Work out the finished part from the listing and answer in its coordinate system (mm). A direction names the side the tool comes from. Round coordinates to 2 decimals unless told otherwise and drop trailing zeros. Write each loop counter-clockwise with the first axis right and the second up, starting at its lowest first coordinate (ties: lowest second). Pieces come first, ordered by that corner, then holes. Notation, with made-up numbers: (-24, 84.25) - (-3, 84.25) arc R33 cw to (-3, 117.25) - close; hole circle Ø6 at (65.5, 21.25). An arc over 180 degrees is marked (long way). Answer as a JSON object with one key per item and string values.
```python
from build123d import *

# Parameters (mm, degrees)
BOSS_EXTRUDE1_DEPTH     = 640
BOSS_EXTRUDE2_DEPTH     = 63
BOSS_EXTRUDE3_DEPTH     = 7
SKETCH26_R              = 6
CUT_EXTRUDE2_DEPTH      = 10
CUT_EXTRUDE1_DEPTH      = 10
CUT_EXTRUDE1_DEPTH_BACK = 10
SKETCH28_R              = 6


with BuildPart() as part:
    # Sketch1 → Boss-Extrude1 (new body)
    with BuildSketch(Plane.XY):
        Polygon((0, 0), (0, 70), (70, 70), (70, 63), (7, 63), (7, 0), align=None)
    extrude(amount=BOSS_EXTRUDE1_DEPTH)

    # Sketch23 → Boss-Extrude2 (add)
    with BuildSketch(Plane(origin=(0, 0, 0), x_dir=(1, 0, 0), z_dir=(0, 1, 0))):
        Polygon((0, -640), (42.5, -713.612159322), (48.562177826, -710.112159322), (7, -640), align=None)
    extrude(amount=BOSS_EXTRUDE2_DEPTH)

    # Sketch25 → Boss-Extrude3 (add)
    with BuildSketch(Plane(origin=(0, 63, 0), x_dir=(1, 0, 0), z_dir=(0, 1, 0))):
        Polygon((70, -640), (0, -640), (42.5, -713.612159322), (70, -713.612159322), align=None)
    extrude(amount=BOSS_EXTRUDE3_DEPTH)

    # Sketch26 → Cut-Extrude2 (cut)
    with BuildSketch(Plane(origin=(-275.556719825, 0, 163.348804279), x_dir=(-0.5099316128113042, 0, -0.8602149442178172), z_dir=(0.8602149442178172, 0, -0.5099316128113042))):
        with Locations((-614.36248118, 31.5)):
            Circle(SKETCH26_R)
        with Locations((-575.357085589, 31.5)):
            Circle(SKETCH26_R)
    extrude(amount=-CUT_EXTRUDE2_DEPTH, mode=Mode.SUBTRACT)

    # Mirror1: part across plane


with BuildPart() as part_1:
    add(part.part)
    add(part.part.mirror(Plane.XY))

    # Sketch28 → Cut-Extrude1 (cut, two sides: drawn at the far end of the back side and taken through both)
    with BuildSketch(Plane(origin=(0, 70, 0), x_dir=(1, 0, 0), z_dir=(0, 1, 0)).offset(-CUT_EXTRUDE1_DEPTH_BACK)):
        with Locations(Location((35, -500, 0), (0, 0, 90))):
            Circle(SKETCH28_R)
        with Locations(Location((35, -165, 0), (0, 0, 90))):
            Circle(SKETCH28_R)
        with Locations(Location((35, 170, 0), (0, 0, 90))):
            Circle(SKETCH28_R)
    extrude(amount=CUT_EXTRUDE1_DEPTH + CUT_EXTRUDE1_DEPTH_BACK, mode=Mode.SUBTRACT)


solid = part_1.part
```
Item 1: For faces 4 (the flat face through (28.072, 31.059, -675.547)), 5 (the flat face through (35, 70, 10)), determine the directions among +Z, -Z, +X, -X, +Y, -Y from which every point of the face is accessible in a straight line to the end or side of a thin tool.
Results found:
{"face 4": "+X, -Y", "face 5": "+Z, -Z, +X, -X, +Y"}
Item 2: Determine the mould class of faces 1 (the flat face through (6, 0, 3)), 2 (the flat face through (28.072, 31.059, 675.547)), 3 (the flat face through (20.95, 34.51, -676.29)) for opening direction Z: pulls with the +Z half, pulls with the -Z half, needs draft (parallel to the pull), parting line crosses it, or undercut.
Results found:
{"face 1": "needs draft", "face 2": "undercut", "face 3": "pulls with the -Z half"}
Item 3: Each of these flat-tipped pins is pushed along its axis until it touches: P1, Ø4, axis at x = 22, y = 50, coming from the +Z side; P2, Ø19, axis at x = 35, z = 284, coming from the -Y side; P3, Ø3, axis at x = 15, y = 50, coming from the +Z side; P4, Ø9.5, axis at x = 35, z = 500, coming from the -Y side. Where does it stop, or does it pass through?
Results found:
{"P1": "z = 681.57", "P2": "y = 63", "P3": "z = 668.58", "P4": "through"}
Item 4: A cutting plane is placed at A-A (z = -202.5). Write down the section's boundary in (x, y), and give its area (3 significant figures).
Results found:
{"outline": "(0, 0) - (7, 0) - (7, 63) - (70, 63) - (70, 70) - (0, 70) - close", "area": "931 mm²"}
Item 5: Consider line 1 along X through (y, z) = (66.75, 165); line 2 along Y through (x, z) = (48.5, -37); line 3 along X through (y, z) = (36.5, -415). Determine where each line is inside the solid, lowest interval first.
Results found:
{"line 1": "0 to 29, 41 to 70", "line 2": "63 to 70", "line 3": "0 to 7"}
